CAD build for the part. Positions are in the model's coordinates, mm. A direction names the side the tool comes from. Coordinates: 2 decimals unless noted, no trailing zeros. Write each loop counter-clockwise with the first axis right and the second up, starting at its lowest first coordinate (ties: lowest second). Pieces come first, ordered by that corner, then holes. Notation, with made-up numbers: M -19.75,10.25 L 27.25,10.25 A24 cw 27.25,44.25 Z; hole C -28.75,2.5 d6. An arc over 180 degrees is marked long. Put each result on its own line as item: value. Start each with the question number.
```python
from build123d import *

# Parameters (mm, degrees)
CROQUIS2_R              = 6
SALIENTE_EXTRUIR1_DEPTH = 12.5
SALIENTE_EXTRUIR2_DEPTH = 15
CROQUIS5_R              = 11.5
CROQUIS5_R_2            = 6
CORTAR_EXTRUIR2_DEPTH   = 5
CROQUIS6_W              = 5
CROQUIS6_H              = 10
SALIENTE_EXTRUIR3_DEPTH = 8
CROQUIS7_R              = 1.7
CORTAR_EXTRUIR3_DEPTH   = 15
CROQUIS8_R              = 5
SALIENTE_EXTRUIR4_DEPTH = 4


with BuildPart() as part:
    # Croquis2 → Saliente-Extruir1 (new body, symmetric)
    with BuildSketch(Plane(origin=(0, 0, 0), x_dir=(0, 0, -1), z_dir=(1, 0, 0))):
        Circle(CROQUIS2_R)
    extrude(amount=SALIENTE_EXTRUIR1_DEPTH, both=True)

    # Croquis3 → Saliente-Extruir2 (add)
    with BuildSketch(Plane.ZY.offset(12.5)):
        Polygon((-15.6, -6), (-6, -6), (-6, 0), (6, 0), (6, -6), (15.6, -6), (15.6, -16), (-15.6, -16), align=None)
    extrude(amount=-SALIENTE_EXTRUIR2_DEPTH)

    # Croquis5 → Cortar-Extruir2 (cut)
    with BuildSketch(Plane(origin=(2.5, 0, 0), x_dir=(0, 0, -1), z_dir=(1, 0, 0))):
        Circle(CROQUIS5_R)
        Circle(CROQUIS5_R_2, mode=Mode.SUBTRACT)
    extrude(amount=-CORTAR_EXTRUIR2_DEPTH, mode=Mode.SUBTRACT)

    # Croquis6 → Saliente-Extruir3 (add)
    with BuildSketch(Plane.ZY.offset(12.5)):
        with Locations((5, -21)):
            Rectangle(CROQUIS6_W, CROQUIS6_H)
        with Locations((-5, -21)):
            Rectangle(CROQUIS6_W, CROQUIS6_H)
    extrude(amount=-SALIENTE_EXTRUIR3_DEPTH)

    # Croquis7 → Cortar-Extruir3 (cut)
    with BuildSketch(Plane.XY.offset(7.5)):
        with Locations((-8.5, -22.3)):
            Circle(CROQUIS7_R)
    extrude(amount=-CORTAR_EXTRUIR3_DEPTH, mode=Mode.SUBTRACT)

    # Croquis8 → Saliente-Extruir4 (add, symmetric)
    with BuildSketch(Plane.XY.offset(15.6)):
        with Locations((-5, -6)):
            Circle(CROQUIS8_R)
    saliente_extruir4 = extrude(amount=SALIENTE_EXTRUIR4_DEPTH, both=True)

    # Simetría1: Saliente-Extruir4 across plane
    add(saliente_extruir4.mirror(Plane.XY))


solid = part.part
```
(1) Slice it at B-B, the plane y = -22.3. Write the cut outline in (x, z), then the cut area to 3 significant figures.
(2) Slice it at D-D, the plane x = -8. State how many separate pieces and enclosed holes the cut face has, then the cut area to 3 significant figures.
(3) Two-plate mould, pull along Y, no slides. Class faces 1 (the face through (-2.5, -8, 0)), 2 (the face through (-5.651, -1.043, 16.545)), 3 (the face through (-9, -20, 7.5)): +Y half, -Y half, draft (parallel to the pull), parting line (faces both ways), or undercut.
(4) Drill centre lines: line 1 (Z direction, x = -6.25, y = -3); line 2 (Y direction, x = -8.5, z = 6.1); line 3 (X direction, y = -15.5, z = -13.5). Where is each one in solid material? Low to high. Write a range as [from, to].
(5) Slice it at C-C, the plane x = -5. Write the cut outline in (y, z), then the cut area to 3 significant figures.
(6) Drop flat-ended pins along their axis: pin 1 (4 mm diameter, centred on y = -23.5, z = 4, fed in from +X); pin 2 (3 mm diameter, centred on x = -6, y = -13.5, fed in from -Z); pin 3 (2.5 mm diameter, centred on x = -8.5, y = -23.5, fed in from -Z). Give the stop position or say it passes through.
(7) Slice it at A-A, the plane y = -17.5. Write the cut outline in (x, z).
(8) Which spindle directions (+Z, -Z, +X, -X, +Y, -Y) get a long thin tool onto all of the face, cutting with end or side? Do faces 4 (the face through (2.95, 5.95, 0.78)), 5 (the face through (-5, -12, 15.6)), 6 (the face through (-9, -20, 2.5)), 7 (the face through (-9, -20, -7.5)). Say none if no direction does.
Result set:
1. outline: M -12.5,-7.5 L -10.2,-7.5 L -10.2,-2.5 L -12.5,-2.5 Z; M -12.5,2.5 L -10.2,2.5 L -10.2,7.5 L -12.5,7.5 Z; M -6.8,-7.5 L -4.5,-7.5 L -4.5,-2.5 L -6.8,-2.5 Z; M -6.8,2.5 L -4.5,2.5 L -4.5,7.5 L -6.8,7.5 Z
1. area: 46.0 mm^2
2. separate pieces: 3
2. enclosed holes: 0
2. area: 604 mm^2
3. face 1: undercut
3. face 2: parting line
3. face 3: draft
4. line 1: z = [-19.6, -11.6], [-6, 6], [11.6, 19.6]
4. line 2: y = [-26, -24], [-20.6, -6]
4. line 3: x = [-12.5, 2.5]
5. outline: M -26,-7.5 L -16,-7.5 L -16,-15.6 L -11,-15.6 L -11,-19.6 L -1,-19.6 L -1,-11.6 L -6,-11.6 L -6,-6 L 0,-6 A6 ccw 0,6 L -6,6 L -6,11.6 L -1,11.6 L -1,19.6 L -11,19.6 L -11,15.6 L -16,15.6 L -16,7.5 L -26,7.5 L -26,2.5 L -16,2.5 L -16,-2.5 L -26,-2.5 Z
5. area: 661 mm^2
6. pin 1: stops at x = -4.5
6. pin 2: stops at z = -15.6
6. pin 3: stops at z = -7.5
7. outline: M -12.5,-7.5 L -4.5,-7.5 L -4.5,-2.5 L -12.5,-2.5 Z; M -12.5,2.5 L -4.5,2.5 L -4.5,7.5 L -12.5,7.5 Z
8. face 4: +X
8. face 5: +Z, -Y
8. face 6: +X, -X, -Y
8. face 7: -Z, +X, -X, -Y
